Study the drawing (mm; zero at the part's minimum x, y, z) and answer. Give positions to 0.01 mm unless a question says otherwise; leave off trailing zeros. Loops run counter-clockwise (first coordinate to the right, second up) from the corner with the lowest first, then second, coordinate; pieces in that order, holes last. Notation, with made-up numbers: (-7.5, 72) - (9.5, 72) arc R9 ccw to (9.5, 81) - close; hole circle Ø5 at (-28.5, 2). An arc over 180 degrees is marked (long way). Use one line per item in the form item = value. Start each with the question number.
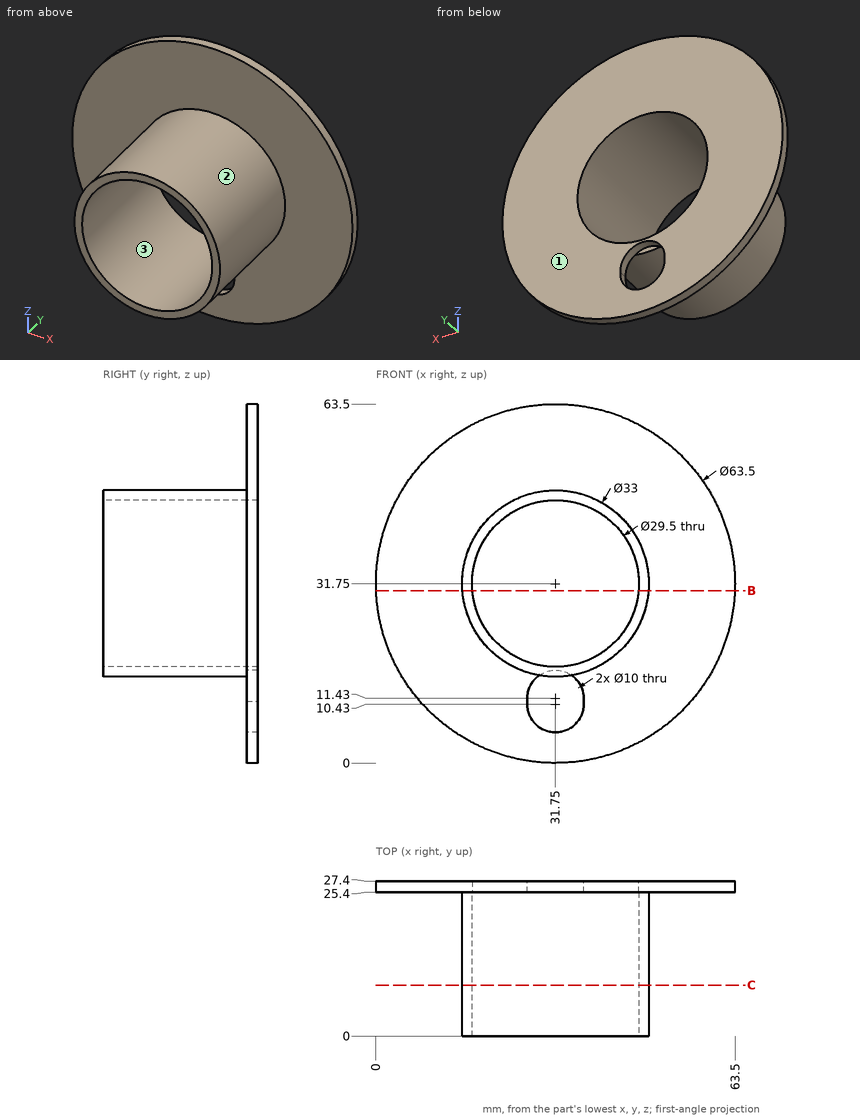
1) Flat-ended cylindrical pins translate along their axes: pin 1 Ø3 at (x, y) = (36, 6) entering from +Z; pin 2 Ø12 at (x, y) = (42, 16.5) entering from -Z; pin 3 Ø4 at (y, z) = (22.5, 49) entering from +X. Find the tip coordinate at first contact, or state that the pin passes through.
2) Find the intervals of material crossed by probe 1 along Z at (x, y) = (31.75, 26.75); probe 2 along Z at (x, y) = (31.75, 14.75), in increasing order.
3) A cutting plane is placed at B-B (z = 30.5). Give the vertices of the cut face in (x, y).
4) Determine the mould class of the marked faces 1, 2 and 3 for opening direction Z: released by +Z, released by -Z, zero draft, split by the parting line, or undercut.
5) A cutting plane is placed at C-C (y = 9). Give the vertices of the cut face in (x, z).
Answer sheet:
q1.pin_1 = 48.02
q1.pin_2 = 15.81
q1.pin_3 = 38.05
q2.probe_1 = 0 to 5.43, 16.43 to 17, 46.5 to 63.5
q2.probe_2 = 15.25 to 17, 46.5 to 48.25
q3.outline = (0.02, 25.4) - (15.3, 25.4) - (15.3, 0) - (17.05, 0) - (17.05, 27.4) - (0.02, 27.4) - close; (46.45, 0) - (48.2, 0) - (48.2, 25.4) - (63.48, 25.4) - (63.48, 27.4) - (46.45, 27.4) - close
q4.face_1 = zero draft
q4.face_2 = split by the parting line
q4.face_3 = undercut
q5.outline = circle Ø33 at (31.75, 31.75); hole circle Ø29.5 at (31.75, 31.75)
